The model under review builds one solid part; all positions refer to its coordinate system, in mm. A direction names the side the tool comes from. Round coordinates to 2 decimals unless told otherwise and drop trailing zeros. Write each loop counter-clockwise with the first axis right and the second up, starting at its lowest first coordinate (ties: lowest second). Pieces come first, ordered by that corner, then holes. Notation, with made-up numbers: M 20,31.5 L 69,31.5 A29 ccw 69,54.5 Z; hole C 61,-20.75 d7. An arc over 180 degrees is marked long. One line per item, written item: value. Start each with the question number.
1) Take a section at B-B, the plane x = 205. Write out the cut boundary in (y, z), and give its area (3 significant figures).
2) Wall thickness on probe 1 along X at (y, z) = (41, -14.5); probe 2 along Y at (x, z) = (-43.5, -1); probe 3 along Z at (x, y) = (245, 80): over which ranges is each line inside the solid? List them lowest first.
3) Tool access review of faces 1 (the face through (-381, 4, 0)), 2 (the face through (5, -32.89, -1)), 3 (the face through (381, 4, 0)), 4 (the face through (5, 42.498, -1)): name each direction out of +Z, -Z, +X, -X, +Y, -Y from which nothing blocks a thin tool from reaching the whole face with its end or side.
4) Take a section at A-A, the plane y = 7. Write out the cut boundary in (x, z), and give its area (3 significant figures).
5) Take a section at C-C, the plane z = 18. Write out the cut boundary in (x, y), and give its area (3 significant figures).
6) Take a section at D-D, the plane x = -388.5. Write out the cut boundary in (y, z).
7) For P1, Ø3, axis at y = 36.5, z = 11, coming from the -X side; P2, Ø21.5, axis at x = -80, z = -9, coming from the +Y side; P3, Ø21.5, axis at y = 17.5, z = -5.5, coming from the +X side, all flat-tipped, find the tip position at first contact; note any pin that passes through.
from build123d import *

# Parameters (mm, degrees)
F0_W     = 75.3882750869
F0_H     = 72.0623135567
F1_DEPTH = 381
F2_W     = 884.8471343517
F2_H     = 169.3414449692
F3_DEPTH = 25.4


with BuildPart() as f1:
    # F0 (on Right) → F1 (new body, symmetric)
    with BuildSketch(Plane.YZ):
        with Locations((4.8041529953, -0.1847893)):
            Rectangle(F0_W, F0_H)
    extrude(amount=F1_DEPTH, both=True)

    # F2 (on face) → F3 (join)
    with BuildSketch(Plane(origin=(0, 0, -36.2159460783), x_dir=(1, 0, 0), z_dir=(0, 0, -1))):
        with Locations((-1.0705441236, -14.7237181664)):
            Rectangle(F2_W, F2_H)
    extrude(amount=F3_DEPTH)


solid = f1.part
Checked values:
1. outline: M -69.95,-61.62 L 99.39,-61.62 L 99.39,-36.22 L 42.5,-36.22 L 42.5,35.85 L -32.89,35.85 L -32.89,-36.22 L -69.95,-36.22 Z
1. area: 9,730 mm2
2. probe 1: x = -381 to 381
2. probe 2: y = -32.89 to 42.5
2. probe 3: z = -61.62 to -36.22
3. face 1: +Z, -X, +Y, -Y
3. face 2: +Z, +X, -X, -Y
3. face 3: +Z, +X, +Y, -Y
3. face 4: +Z, +X, -X, +Y
4. outline: M -443.49,-61.62 L 441.35,-61.62 L 441.35,-36.22 L 381,-36.22 L 381,35.85 L -381,35.85 L -381,-36.22 L -443.49,-36.22 Z
4. area: 77,400 mm2
5. outline: M -381,-32.89 L 381,-32.89 L 381,42.5 L -381,42.5 Z
5. area: 57,400 mm2
6. outline: M -69.95,-61.62 L 99.39,-61.62 L 99.39,-36.22 L -69.95,-36.22 Z
7. P1: stops at x = -381
7. P2: stops at y = 42.5
7. P3: stops at x = 381
